from build123d import *

# Parameters (mm, degrees)
SKETCH1_R           = 2.5
BOSS_EXTRUDE1_DEPTH = 20
FILLET1_R           = 10
SKETCH2_R           = 1.5
CUT_EXTRUDE1_DEPTH  = 20
SKETCH3_R           = 2.5
CUT_EXTRUDE2_DEPTH  = 10
FILLET2_R           = 10


with BuildPart() as part:
    # Sketch1 → Boss-Extrude1 (new body)
    with BuildSketch(Plane.XY):
        with BuildLine():
            Line((52.5, 20.781588347), (249, 20.781588347))
            Line((249, 20.781588347), (249, -124.218411653))
            Line((249, -124.218411653), (-249, -124.218411653))
            Line((-249, -124.218411653), (-249, 20.781588347))
            Line((-249, 20.781588347), (-52.5, 20.781588347))
            Line((-52.5, 20.781588347), (-52.5, -31.718411653))
            ThreePointArc((-52.5, -31.718411653), (0, -84.218411653), (52.5, -31.718411653))
            Line((52.5, -31.718411653), (52.5, 20.781588347))
        make_face()
        with Locations((-163.25, -116.718411653)):
            Circle(SKETCH1_R, mode=Mode.SUBTRACT)
        with Locations((-153.25, -116.718411653)):
            Circle(SKETCH1_R, mode=Mode.SUBTRACT)
        with Locations((211.75, -116.718411653)):
            Circle(SKETCH1_R, mode=Mode.SUBTRACT)
        with Locations((221.75, -116.718411653)):
            Circle(SKETCH1_R, mode=Mode.SUBTRACT)
    extrude(amount=BOSS_EXTRUDE1_DEPTH)

    # Fillet1
    fillet1_edges = [part.edges().sort_by_distance(p)[0] for p in [
        (249, -124.218411653, 10),
        (-249, -124.218411653, 10),
    ]]
    fillet(fillet1_edges, radius=FILLET1_R)

    # Sketch2 → Cut-Extrude1 (cut)
    with BuildSketch(Plane.XY.offset(20)):
        with Locations((-177.282485579, -58.435926074)):
            Circle(SKETCH2_R)
        with Locations((-190.717514421, -45.000897232)):
            Circle(SKETCH2_R)
        with Locations((190.717514421, -45.000897232)):
            Circle(SKETCH2_R)
        with Locations((177.282485579, -58.435926074)):
            Circle(SKETCH2_R)
    extrude(amount=-CUT_EXTRUDE1_DEPTH, mode=Mode.SUBTRACT)

    # Sketch3 → Cut-Extrude2 (cut)
    with BuildSketch(Plane(origin=(0, 20.781588347, 0), x_dir=(1, 0, 0), z_dir=(0, 1, 0))):
        with Locations(Location((-199, -10, 0), (0, 0, 180))):
            Circle(SKETCH3_R)
        with Locations(Location((-102.5, -10, 0), (0, 0, 180))):
            Circle(SKETCH3_R)
        with Locations((102.5, -10)):
            Circle(SKETCH3_R)
        with Locations((199, -10)):
            Circle(SKETCH3_R)
    extrude(amount=-CUT_EXTRUDE2_DEPTH, mode=Mode.SUBTRACT)

    # Fillet2
    fillet2_edges = [part.edges().sort_by_distance(p)[0] for p in [
        (-249, 20.781588347, 10),
        (-52.5, 20.781588347, 10),
        (52.5, 20.781588347, 10),
        (249, 20.781588347, 10),
    ]]
    fillet(fillet2_edges, radius=FILLET2_R)


solid = part.part
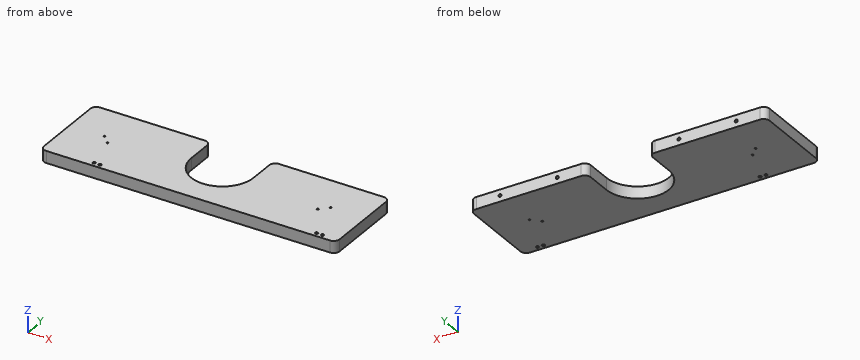
Part model, mm, in its own coordinate system. Give positions to 0.01 mm unless a question says otherwise; leave off trailing zeros. Loops run counter-clockwise (first coordinate to the right, second up) from the corner with the lowest first, then second, coordinate; pieces in that order, holes last. Notation, with made-up numbers: (6, 29) -> (14, 29) arc R20 cw to (14, 52) -> close; hole circle Ø8 at (23, 64.25). An arc over 180 degrees is marked (long way). Write each question's results on one line, items separated by ' | '. Start each with the question number.
Q1. Band-saw the part on B-B on z = 17. Count the separate pieces of the cut face and the enclosed holes in it, plus the area to 3 significant figures.
Q2. Band-saw the part on A-A on y = -20.5. List the corners of the cut face in (x, z).
Q3. Wall check: L1, parallel to X at y = -1.5, z = 10.75; L2, parallel to X at y = -114.5, z = 7.75; L3, parallel to Y at x = 221.75, z = 6.25. Give the ranges that are in metal, low to high.
Q4. Band-saw the part on C-C on x = 34. List the corners of the cut face in (y, z), plus the area to 3 significant figures.
Q5. Pin check, flat tips, straight feed: P1, Ø3, axis at x = -163.25, y = -116.72, coming from the -Z side; P2, Ø4.5, axis at x = 199, z = 10, coming from the +Y side; P3, Ø3, axis at x = -10, z = 15, coming from the +Y side. Stop position of each tip, or through.
Results are:
1) separate pieces: 1 | enclosed holes: 8 | area: 62,100 mm²
2) outline: (-249, 0) -> (-52.5, 0) -> (-52.5, 20) -> (-249, 20) -> close; (52.5, 0) -> (249, 0) -> (249, 20) -> (52.5, 20) -> close
3) L1: x = -249 to -52.5, 52.5 to 249 | L2: x = -249 to -164.4, -162.1 to -154.4, -152.1 to 210.6, 212.9 to 220.6, 222.9 to 249 | L3: y = -124.22 to -119.22, -114.22 to 20.78
4) outline: (-124.22, 0) -> (-71.72, 0) -> (-71.72, 20) -> (-124.22, 20) -> close | area: 1,050 mm²
5) P1: passes through | P2: stops at y = 10.78 | P3: stops at y = -82.94
